Check sheet for the drawn part. Datum: minimum x, y, z corner. Units: mm. A direction names the side the tool comes from. Round coordinates to 2 decimals unless told otherwise and drop trailing zeros. Write each loop counter-clockwise with the first axis right and the second up, starting at its lowest first coordinate (ties: lowest second). Pieces come first, ordered by that corner, then holes. Notation, with made-up numbers: M -20.75,40.25 L 0.25,40.25 A23 ccw 0.25,51.25 Z; hole C -20,50 d3. An arc over 180 degrees is marked long. Answer in a Markdown table with one row per item. Add a question column.
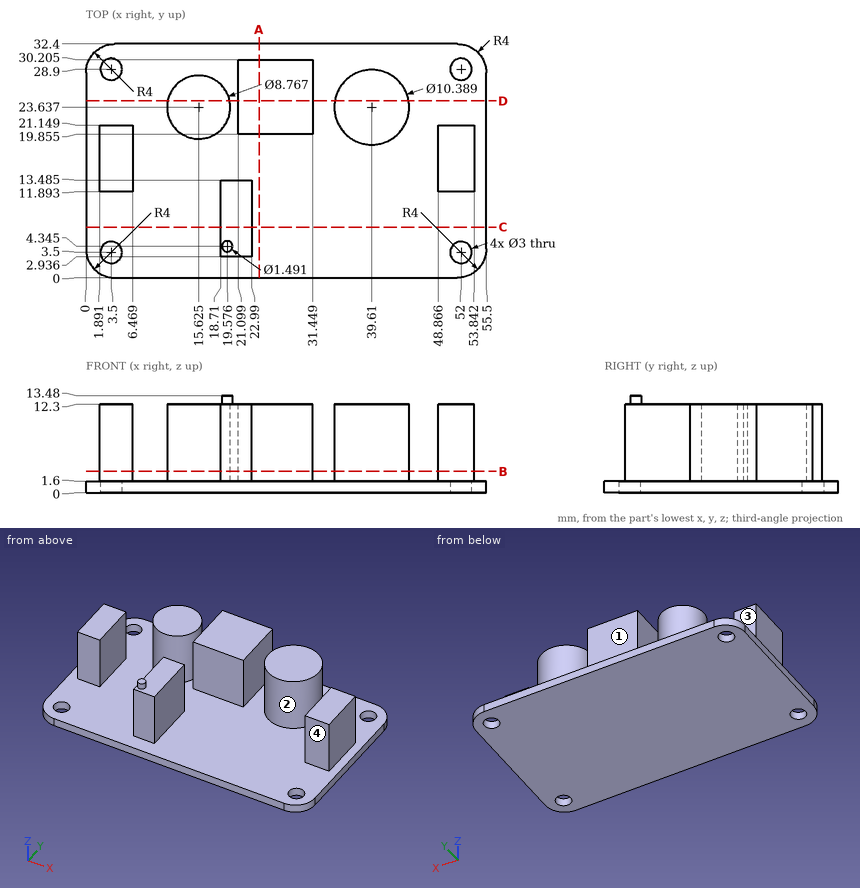
Item 1: Section check C-C, the plane y = 7. Record the boundary of the cut face in (x, z).
Item 2: Section check A-A, the plane x = 24. Record the boundary of the cut face in (y, z) (1 decimal).
Item 3: Gauge pin test, flat ends, axial feed: pin 1 Ø2.5 at (x, z) = (51.5, 5) entering from -Y; pin 2 Ø5 at (x, y) = (3, 14) entering from +Z; pin 3 Ø3 at (y, z) = (17.5, 8.5) entering from +X; pin 4 Ø1.8 at (x, y) = (3.5, 3.5) entering from +Z. Record the tip position at first contact, or that the pin passes through.
Item 4: Scan lines: probe 1 along Y at (x, z) = (52, 1); probe 2 along Y at (x, z) = (29, 1.75) (1 decimal); probe 3 along Z at (x, y) = (9, 24). Record each from-to range of solid material in increasing order. Write a range as from..to.
Item 5: Access from +Z, -Z, +X, -X, +Y, -Y to the whole of each face (thin tool, end or side, straight path). Record for the marked faces 1, 2, 3 and 4.
Item 6: Section check D-D, the plane y = 24.5. Record the boundary of the cut face in (x, z).
Item 7: Section check B-B, the plane z = 3. Give the number of separate pieces and of enclosed holes in the cut face, and give its area (3 significant figures).
Result sheet:
| question | item | result |
|---|---|---|
| 1 | outline | M 0,0 L 55.5,0 L 55.5,1.6 L 22.99,1.6 L 22.99,12.3 L 18.71,12.3 L 18.71,1.6 L 0,1.6 Z |
| 2 | outline | M 0,0 L 32.4,0 L 32.4,1.6 L 30.2,1.6 L 30.2,12.3 L 19.9,12.3 L 19.9,1.6 L 0,1.6 Z |
| 3 | pin 1 | stops at y = 11.89 |
| 3 | pin 2 | stops at z = 12.3 |
| 3 | pin 3 | stops at x = 53.84 |
| 3 | pin 4 | passes through |
| 4 | probe 1 | y = 0.03..2, 5..27.4, 30.4..32.37 |
| 4 | probe 2 | y = 19.9..30.2 |
| 4 | probe 3 | z = 0..1.6 |
| 5 | face 1 | +Z, +X, -X, +Y |
| 5 | face 2 | +Z |
| 5 | face 3 | +Z, -X, +Y |
| 5 | face 4 | +Z, +X, -Y |
| 6 | outline | M 0,0 L 55.5,0 L 55.5,1.6 L 44.73,1.6 L 44.73,12.3 L 34.49,12.3 L 34.49,1.6 L 31.45,1.6 L 31.45,12.3 L 21.1,12.3 L 21.1,1.6 L 19.92,1.6 L 19.92,12.3 L 11.33,12.3 L 11.33,1.6 L 0,1.6 Z |
| 7 | separate pieces | 6 |
| 7 | enclosed holes | 0 |
| 7 | area | 386 mm^2 |
